Autodesk Inventor part; units mm, degrees
ref_plane "YZ Plane" through (0, 0, 0) normal (1, 0, 0) x (0, 1, 0)
ref_plane "XZ Plane" through (0, 0, 0) normal (0, 1, 0) x (-1, 0, 0)
ref_plane "XY Plane" through (0, 0, 0) normal (0, 0, 1) x (1, 0, 0)
sketch "Sketch1" plane through (0, 0, 0) normal (0, 0, 1) x (1, 0, 0)
  circle A0 centre (0, 0) radius 4.5
  dimension "d0" = 9
extrude "Extrusion1" add sketch "Sketch1" along normal blind 3.5
fillet "Fillet1" radius 3 1 edges at (-4.5, 0, 3.5)
sketch "Sketch2" plane through (0, 0, 3.5) normal (0, 0, 1) x (1, 0, 0)
  line L0 (1.7321, 0) -> (0.866, -1.5)
  line L1 (0.866, -1.5) -> (-0.866, -1.5)
  line L2 (-0.866, -1.5) -> (-1.7321, 0)
  line L3 (-1.7321, 0) -> (-0.866, 1.5)
  line L4 (-0.866, 1.5) -> (0.866, 1.5)
  line L5 (0.866, 1.5) -> (1.7321, 0)
  point P0 (0, 0)
  point P1 (0, 0)
  dimension "d4" = 3
extrude "Extrusion2" cut sketch "Sketch2" against normal blind 1.5
properties part number "ENDER 3 E_PLATE_SCREW" material "Steel, High Strength, Low Alloy"
Source: CAD feature listing. Evaluate the final solid. Frame: model axes, mm. Give positions to 0.01 mm unless a question says otherwise; leave off trailing zeros. Write item = value, one per line.
Q1. First-contact query: pin 1 (1.5 mm diameter, centred on y = -1.5, z = 3, fed in from -X); pin 2 (1.5 mm diameter, centred on y = 0.5, z = 1.5, fed in from +X); pin 3 (1.7 mm diameter, centred on x = -0.5, z = 2.5, fed in from +Y). Flat tips, straight axial feed; report the tip coordinate or a pass-through.
Here are the results:
pin_1 = -3.7
pin_2 = 4.48
pin_3 = 4.25
Q2. Mould query, pull axis Y, two halves, no side actions, for faces 1 (the face through (0, 0, 2)), 2 (the face through (0, 0, 0)), 3 (the face through (-0.59, -4.46, 0.25)). Classes: +Y half, -Y half, draft (parallel to the pull), parting line (faces both ways), or undercut.
Here are the results:
face_1 = undercut
face_2 = draft
face_3 = parting line
Q3. Line query: line 1 (Y direction, x = 1, z = 2.45); line 2 (X direction, y = -1, z = 2.85); line 3 (Y direction, x = -0.5, z = 2.7). Output: solid intervals per line, ascending. Write a range as from..to.
Here are the results:
line_1 = -3.65..-1.27, 1.27..3.65
line_2 = -3.21..-1.15, 1.15..3.21
line_3 = -3.5..-1.5, 1.5..3.5
